from build123d import *

# Parameters (mm, degrees)
SKETCH1_W               = 80
SKETCH1_H               = 80
SKETCH1_R               = 3
BOSS_EXTRUDE1_DEPTH     = 150
SKETCH2_W               = 50
SKETCH2_H               = 80
CUT_EXTRUDE1_DEPTH      = 80
SKETCH3_R               = 3
CUT_EXTRUDE2_DEPTH      = 1
CUT_EXTRUDE2_DEPTH_BACK = 81
FILLET1_R               = 10


with BuildPart() as part:
    # Sketch1 → Boss-Extrude1 (new body)
    with BuildSketch(Plane(origin=(0, 0, 0), x_dir=(1, 0, 0), z_dir=(0, 1, 0))):
        Rectangle(SKETCH1_W, SKETCH1_H)
        Circle(SKETCH1_R, mode=Mode.SUBTRACT)
    extrude(amount=BOSS_EXTRUDE1_DEPTH)

    # Sketch2 → Cut-Extrude1 (cut)
    with BuildSketch(Plane(origin=(0, 150, 0), x_dir=(1, 0, 0), z_dir=(0, 1, 0))):
        Rectangle(SKETCH2_W, SKETCH2_H)
    extrude(amount=-CUT_EXTRUDE1_DEPTH, mode=Mode.SUBTRACT)

    # Sketch3 → Cut-Extrude2 (cut, two sides)
    with BuildSketch(Plane(origin=(40, 0, 0), x_dir=(0, 0, -1), z_dir=(1, 0, 0))) as cut_extrude2_sk:
        with Locations((0, 110)):
            Circle(SKETCH3_R)
    extrude(amount=CUT_EXTRUDE2_DEPTH, mode=Mode.SUBTRACT)
    extrude(cut_extrude2_sk.sketch, amount=-CUT_EXTRUDE2_DEPTH_BACK, mode=Mode.SUBTRACT)

    # Fillet1
    fillet1_edges = [part.edges().sort_by_distance(p)[0] for p in [
        (-32.5, 150, 40),
        (32.5, 150, 40),
        (-32.5, 150, -40),
        (32.5, 150, -40),
    ]]
    fillet(fillet1_edges, radius=FILLET1_R)


solid = part.part
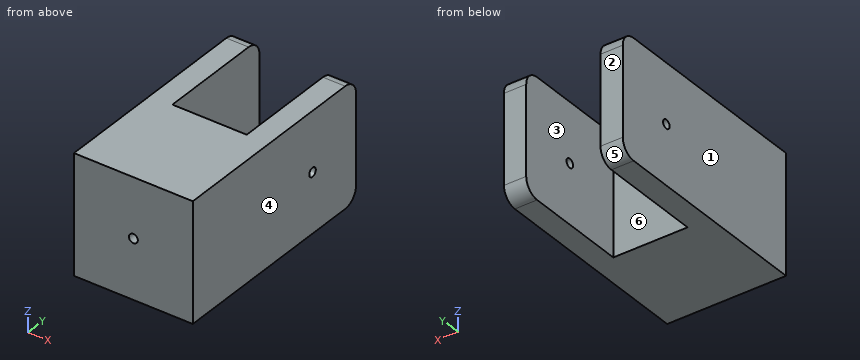
Could you check a few things on this model? Use its own coordinates, in mm. Face numbers are marked on the shaded views. A direction names the side the tool comes from. Coordinates: 2 decimals unless noted, no trailing zeros. Loops run counter-clockwise (first coordinate to the right, second up) from the corner with the lowest first, then second, coordinate; pieces in that order, holes last. Notation, with made-up numbers: (15, 65.5) -> (62, 65.5) arc R30 cw to (62, 93.5) -> close; hole circle Ø1 at (-29, 45). An arc over 180 degrees is marked (long way). Answer in a Markdown table with one row per item.
(1) For the marked faces 5 and 6, which set-ups out of +Z, -Z, +X, -X, +Y, -Y let a thin tool reach every point of the face, with its end or its side?
Results found:
| item | result |
|---|---|
| face 5 | -Z, +X, -X, +Y |
| face 6 | +Z, -Z, +Y |
(2) Imagine slicing it at B-B (z = 0). List the corners of the cut face in (x, y) for me, plus the area to 3 significant figures.
Results found:
| item | result |
|---|---|
| outline | (-40, 0) -> (-3, 0) -> (-3, 70) -> (-25, 70) -> (-25, 107) -> (-40, 107) -> close; (-40, 113) -> (-25, 113) -> (-25, 150) -> (-40, 150) -> close; (3, 0) -> (40, 0) -> (40, 107) -> (25, 107) -> (25, 70) -> (3, 70) -> close; (25, 113) -> (40, 113) -> (40, 150) -> (25, 150) -> close |
| area | 7,400 mm^2 |
(3) If I drill on probe 1 along X at (y, z) = (101, 36.5); probe 2 along Y at (x, z) = (-29, 0); probe 3 along Y at (x, z) = (-12, -7.5), over which ranges is the centre line in solid material (lowest first)?
Results found:
| item | result |
|---|---|
| probe 1 | x = -40 to -25, 25 to 40 |
| probe 2 | y = 0 to 107, 113 to 150 |
| probe 3 | y = 0 to 70 |
(4) Imagine slicing it at D-D (y = 110). List the corners of the cut face in (x, z) for me.
Results found:
| item | result |
|---|---|
| outline | (-40, -40) -> (-25, -40) -> (-25, -3) -> (-40, -3) -> close; (-40, 3) -> (-25, 3) -> (-25, 40) -> (-40, 40) -> close; (25, -40) -> (40, -40) -> (40, -3) -> (25, -3) -> close; (25, 3) -> (40, 3) -> (40, 40) -> (25, 40) -> close |
(5) Imagine slicing it at C-C (x = 0). List the corners of the cut face in (y, z) for me.
Results found:
| item | result |
|---|---|
| outline | (0, -40) -> (70, -40) -> (70, -3) -> (0, -3) -> close; (0, 3) -> (70, 3) -> (70, 40) -> (0, 40) -> close |
(6) Will these pins go through, and if not, where does the flat tip stop? pin 1 Ø3.5 at (y, z) = (110, 0) entering from -X; pin 2 Ø25 at (x, z) = (-5, 11.5) entering from +Y.
Results found:
| item | result |
|---|---|
| pin 1 | passes through |
| pin 2 | stops at y = 70 |
(7) Imagine slicing it at A-A (y = 76). List the corners of the cut face in (x, z) for me.
Results found:
| item | result |
|---|---|
| outline | (-40, -40) -> (-25, -40) -> (-25, 40) -> (-40, 40) -> close; (25, -40) -> (40, -40) -> (40, 40) -> (25, 40) -> close |
(8) Thinking about a two-plate mould opening in X: for the marked faces 1, 2, 3 and 4, which applies, released by +X, released by -X, zero draft, split by the parting line, or undercut?
Results found:
| item | result |
|---|---|
| face 1 | released by -X |
| face 2 | zero draft |
| face 3 | undercut |
| face 4 | released by +X |
